Input: part model. Units: mm. Frame: model coordinates. A direction names the side the tool comes from. Coordinates: 2 decimals unless noted, no trailing zeros. Order: outer loops, then holes, each group sorted by start corner. A loop starts at its lowest first (then second) coordinate and runs counter-clockwise, first axis right, second up. Notation, with made-up numbers: (-16, 15.25) -> (26, 15.25) arc R9 cw to (26, 26.25) -> close; hole circle Ø6 at (11.5, 64). An arc over 180 degrees is marked (long way). Write each question's results on one line, items separated by ' | '.
Autodesk Inventor part; units mm, degrees
ref_plane "YZ Plane" through (0, 0, 0) normal (1, 0, 0) x (0, 1, 0)
ref_plane "XZ Plane" through (0, 0, 0) normal (0, 1, 0) x (-1, 0, 0)
ref_plane "XY Plane" through (0, 0, 0) normal (0, 0, 1) x (1, 0, 0)
sketch "Sketch1" plane through (0, 0, 0) normal (0, 0, 1) x (1, 0, 0)
  line L0 (0, 0) -> (0, 58)
  line L1 (0, 58) -> (20, 58)
  line L2 (20, 58) -> (20, 0)
  line L3 (20, 0) -> (0, 0)
  line L4 (40, 0) -> (40, 58)
  line L5 (40, 58) -> (55, 68)
  line L6 (55, 68) -> (55, 80.225)
  line L7 (55, 80.225) -> (20, 80.225)
  line L8 (20, 80.225) -> (20, -22.225)
  line L9 (20, -22.225) -> (55, -22.225)
  line L10 (55, -22.225) -> (55, -10)
  line L11 (55, -10) -> (40, 0)
  line L12 (20, 0) -> (8.5, 0)
  line L13 (8.5, 0) -> (8.5, 58)
  line L14 (8.5, 58) -> (20, 58)
  line L15 (20, 58) -> (20, 0)
  line L16 (8.5, -9.725) -> (20, -9.725)
  line L17 (20, -9.725) -> (20, 67.725)
  line L18 (20, 67.725) -> (8.5, 67.725)
  line L19 (8.5, 67.725) -> (8.5, -9.725)
  dimension "d0" = 58
  dimension "d1" = 20
  dimension "d9" = 12.225
  dimension "d10" = 10
  dimension "d14" = 8.5
  dimension "d15" = 102.45
  dimension "d16" = 77.45
  dimension "d17" = 12.5
  dimension "d18" = 35
  dimension "d19" = 40
  dimension "d20" = 35
  dimension "d21" = 12.225
  dimension "d22" = 10
revolve "Revolution1" add sketch "Sketch1" angle 360 about axis through (0, 0, 0) along (0, 1, 0) contours L13 L1 L2 L3 | L3 L8 L16 L19 | L19 L18 L8 L1 | L2 L8 L7 L6 L5 L4 L11 L10 L9
ref_plane "Work Plane1" through (0, 29, 0) normal (0, -1, 0) x (1, 0, 0)
equation "\"d9\" = d5"
equation "\"d10\" = d7"
equation "\"d17\" = -0.5 * d16 + 0.5 * d15"
equation "\"d20\" = d18"
equation "\"d21\" = d9"
properties part number "1219_Middle Roller_V1" material "Wood (Maple)"
(1) Pin query (flat end, axial travel): P1, Ø4, axis at y = -10.5, z = 21, coming from the +X side; P2, Ø12, axis at x = 3, y = -11.5, coming from the -Z side; P3, Ø8, axis at x = 13, z = -5.5, coming from the +Y side (3 decimals). Return the tip coordinate at first contact, or that it passes through.
Return value:
P1: x = 51.61 | P2: z = -55 | P3: y = 67.725
(2) Reachability of faces 1 (the face through (39.048, -0.626, 12.297)), 2 (the face through (-4.336, -16.062, -19.524)), 3 (the face through (-11.923, 74.198, 53.692)), 4 (the face through (9, 67.725, 0)) from +Z, -Z, +X, -X, +Y, -Y: full face, straight path, thin tool, end or side. Return the list, or none.
Return value:
face 1: none | face 2: -Y | face 3: +Y, -Y | face 4: +Y
(3) Cut plane B-B, the plane x = 0. Return loops of the section in (y, z) (3 decimals), plus the area to 3 significant figures.
Return value:
outline: (-22.225, -55) -> (-10, -55) -> (0, -40) -> (58, -40) -> (68, -55) -> (80.225, -55) -> (80.225, -20) -> (67.725, -20) -> (67.725, -8.5) -> (-9.725, -8.5) -> (-9.725, -20) -> (-22.225, -20) -> close; (-22.225, 20) -> (-9.725, 20) -> (-9.725, 8.5) -> (67.725, 8.5) -> (67.725, 20) -> (80.225, 20) -> (80.225, 55) -> (68, 55) -> (58, 40) -> (0, 40) -> (-10, 55) -> (-22.225, 55) -> close | area: 6,910 mm2
(4) Mould query, pull axis Z, two halves, no side actions, for faces 5 (the face through (-1, 80.225, 24)), 6 (the face through (-4.336, 73.887, -19.524)), 7 (the face through (-8.67, 29.41, 39.05)). Classes: +Z half, -Z half, draft (parallel to the pull), parting line (faces both ways), or undercut.
Return value:
face 5: draft | face 6: undercut | face 7: parting line
(5) Cut plane A-A, the plane z = 0. Return loops of the section in (x, y) (3 decimals), plus the area to 3 significant figures.
Return value:
outline: (-55, -22.225) -> (-20, -22.225) -> (-20, -9.725) -> (-8.5, -9.725) -> (-8.5, 67.725) -> (-20, 67.725) -> (-20, 80.225) -> (-55, 80.225) -> (-55, 68) -> (-40, 58) -> (-40, 0) -> (-55, -10) -> close; (8.5, -9.725) -> (20, -9.725) -> (20, -22.225) -> (55, -22.225) -> (55, -10) -> (40, 0) -> (40, 58) -> (55, 68) -> (55, 80.225) -> (20, 80.225) -> (20, 67.725) -> (8.5, 67.725) -> close | area: 6,910 mm2
(6) Line query: line 1 along X through (y, z) = (-14, 0); line 2 along Z through (x, y) = (0, 12); line 3 along Y through (x, z) = (40.5, -2) (3 decimals). Output: solid intervals per line, ascending. Write a range as from..to.
Return value:
line 1: -55..-20, 20..55 | line 2: -40..-8.5, 8.5..40 | line 3: -22.225..-0.366, 58.366..80.225
(7) Cut plane C-C, the plane y = 45. Return loops of the section in (x, z).
Return value:
outline: circle Ø80 at (0, 0); hole circle Ø17 at (0, 0)
